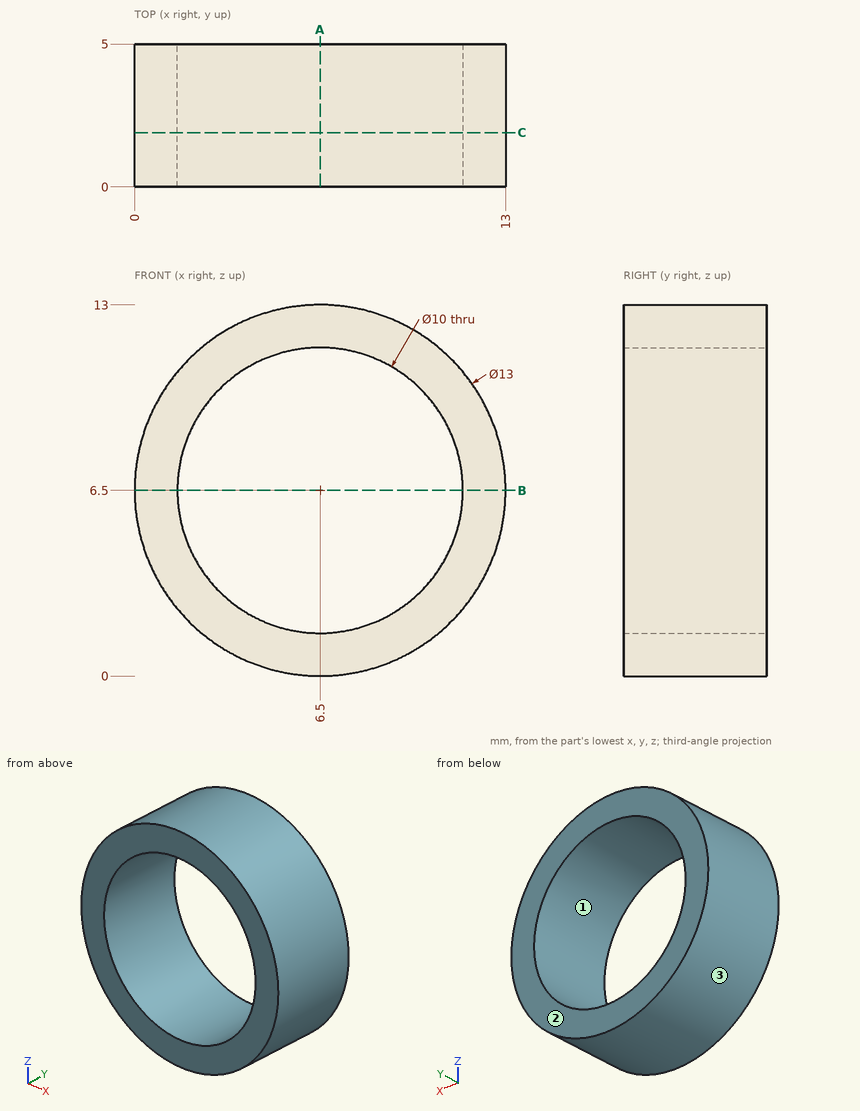
Here's the drawing with two shaded views (mm, measured from the low corner). I have some questions. Coordinates: 2 decimals unless noted, no trailing zeros. Loops run counter-clockwise (first coordinate to the right, second up) from the corner with the lowest first, then second, coordinate; pieces in that order, holes last. Notation, with made-up numbers: M 76.25,48 L 90.25,48 A6 cw 90.25,56 Z; hole C 87.5,-3 d7. An arc over 180 degrees is marked long. Answer as CSV lines item,"result". Start each with the question number.
1. If I drill on probe 1 along Z at (x, y) = (6.5, 1.95); probe 2 along Z at (x, y) = (4.5, 2.6); probe 3 along X at (y, z) = (1.3, 10), over which ranges is the centre line in solid material (lowest first)? Write a range as [from, to].
2. Suppose I cut it at B-B, the plane z = 6.5. List the corners of the cut face in (x, y) for me, plus the area to 3 significant figures.
3. Suppose I cut it at A-A, the plane x = 6.5. List the corners of the cut face in (y, z) for me.
4. For pin 1 Ø1 at (x, y) = (10, 1.5) entering from +Z; pin 2 Ø3 at (y, z) = (1, 10) entering from -X; pin 3 Ø2 at (x, y) = (8.5, 3) entering from -Z; pin 4 Ø6 at (x, z) = (8, 8) entering from -Y, each with a flat end and sliding along its axis, tell me the tip position at first contact or that it passes through.
5. Suppose I cut it at C-C, the plane y = 1.9. List the corners of the cut face in (x, z) for me, plus the area to 3 significant figures.
6. Thinking about a two-plate mould opening in X: for the marked faces 1, 2 and 3, which applies, +X half, -X half, draft (parallel to the pull), parting line (faces both ways), or undercut?
Output:
1,probe 1,"z = [0, 1.5], [11.5, 13]"
1,probe 2,"z = [0.32, 1.92], [11.08, 12.68]"
1,probe 3,"x = [1.02, 2.93], [10.07, 11.98]"
2,outline,"M 0,0 L 1.5,0 L 1.5,5 L 0,5 Z; M 11.5,0 L 13,0 L 13,5 L 11.5,5 Z"
2,area,"15.0 mm^2"
3,outline,"M 0,0 L 5,0 L 5,1.5 L 0,1.5 Z; M 0,11.5 L 5,11.5 L 5,13 L 0,13 Z"
4,pin 1,"stops at z = 12.27"
4,pin 2,"stops at x = 0.32"
4,pin 3,"stops at z = 0.08"
4,pin 4,"stops at y = 0"
5,outline,"C 6.5,6.5 d13; hole C 6.5,6.5 d10"
5,area,"54.2 mm^2"
6,face 1,"undercut"
6,face 2,"draft"
6,face 3,"parting line"
